Source: CAD feature listing. Evaluate the final solid. Frame: model axes, mm. A direction names the side the tool comes from. Coordinates: 2 decimals unless noted, no trailing zeros. Order: outer loops, then holes, each group sorted by start corner. A loop starts at its lowest first (then second) coordinate and runs counter-clockwise, first axis right, second up. Notation, with made-up numbers: (0, -24) - (27, -24) arc R21 ccw to (27, -3) - close; hole circle Ø3 at (34.25, 39). An arc over 180 degrees is marked (long way). One line per question, with ' | ' between items.
Autodesk Inventor part; units mm, degrees
ref_plane "YZ Plane" through (0, 0, 0) normal (1, 0, 0) x (0, 1, 0)
ref_plane "XZ Plane" through (0, 0, 0) normal (0, 1, 0) x (-1, 0, 0)
ref_plane "XY Plane" through (0, 0, 0) normal (0, 0, 1) x (1, 0, 0)
sketch "Skizze1" plane through (0, 0, 0) normal (0, 0, 1) x (1, 0, 0)
  line L0 (0, 0) -> (0, 3.95)
  line L1 (0, 3.95) -> (12, 3.95)
  line L2 (12, 3.95) -> (12, 4)
  line L3 (12, 4) -> (56, 4)
  line L4 (56, 4) -> (56, 5)
  line L5 (56, 5) -> (60.1, 5)
  line L6 (60.1, 5) -> (60.1, 4)
  line L7 (60.1, 4) -> (120.1, 4)
  line L8 (120.1, 4) -> (120.1, 0)
  line L9 (120.1, 0) -> (0, 0)
  dimension "d0" = 3.95
  dimension "d1" = 12
  dimension "d3" = 4
  dimension "d6" = 44
  dimension "d8" = 48.1
  dimension "d9" = 5
  dimension "d10" = 60
revolve "Umdrehung1" add sketch "Skizze1" angle 360 about axis through (120.1, 0, 0) along (-1, 0, 0)
thread "Gewinde1"
chamfer "Fase1" distance 0.8 angle 45 1 edges at (0, -3.95, 0)
chamfer "Fase2" distance 0.3 angle 45 2 edges at (56, -5, 0) (60.1, -5, 0)
properties part number "Welle"
(1) Cut plane A-A (y = 0). Return the cut outline in (x, z).
Taken from the geometry:
outline: (0, -3.15) - (0.8, -3.95) - (12, -3.95) - (12, -4) - (56, -4) - (56, -4.7) - (56.3, -5) - (59.8, -5) - (60.1, -4.7) - (60.1, -4) - (120.1, -4) - (120.1, 4) - (60.1, 4) - (60.1, 4.7) - (59.8, 5) - (56.3, 5) - (56, 4.7) - (56, 4) - (12, 4) - (12, 3.95) - (0.8, 3.95) - (0, 3.15) - close
(2) Material intervals for L1, parallel to X at y = -0.5, z = 4.5; L2, parallel to Z at x = 53, y = 0; L3, parallel to Y at x = 33.5, z = -0.5, sorted ascending. Write a range as from..to.
Taken from the geometry:
L1: x = 56..60.1 | L2: z = -4..4 | L3: y = -3.97..3.97
(3) Cut plane C-C (x = 43). Return the cut outline in (y, z).
Taken from the geometry:
outline: circle Ø8 at (0, 0)
(4) Pin query (flat end, axial travel): P1, Ø1.5, axis at x = 80.5, y = 1.5, coming from the -Z side; P2, Ø6, axis at x = 51.5, y = 1.5, coming from the +Z side; P3, Ø1.5, axis at x = 78, y = -4, coming from the +Z side. Return the tip coordinate at first contact, or that it passes through.
Taken from the geometry:
P1: stops at z = -3.93 | P2: stops at z = 4 | P3: stops at z = 2.33
(5) Set-up query: faces 1 (the flat face through (120.1, 0, 0)), 2 (the cylindrical face through (90.52, -0.867, -3.905)), 3 (the cylindrical face through (6.478, -3.135, -2.404)). Return all of +Z, -Z, +X, -X, +Y, -Y with unobstructed straight access to the full face (end or side cutting, diameter ignored); none if empty.
Taken from the geometry:
face 1: +Z, -Z, +X, +Y, -Y | face 2: +X | face 3: -X
